Part model, mm, in its own coordinate system. A direction names the side the tool comes from. Coordinates: 2 decimals unless noted, no trailing zeros. Write each loop counter-clockwise with the first axis right and the second up, starting at its lowest first coordinate (ties: lowest second). Pieces come first, ordered by that corner, then holes. Notation, with made-up numbers: (57.5, -29) - (61.5, -29) arc R25 cw to (61.5, -13) - close; hole circle Ø8 at (61, 24.5). An arc over 180 degrees is marked (long way). Write each question's results on one line, items separated by ' | '.
from build123d import *

# Parameters (mm, degrees)
SKETCH1_R           = 3.7084
SKETCH1_W           = 1.778
SKETCH1_H           = 1.5875
SKETCH1_W_2         = 1.5875
SKETCH1_H_2         = 1.3208
BOSS_EXTRUDE1_DEPTH = 1.5875
SKETCH3_W           = 3.683
SKETCH3_H           = 3.302
CUT_EXTRUDE1_DEPTH  = 23.34938408
FILLET1_R           = 1.27


with BuildPart() as part:
    # Sketch1 → Boss-Extrude1 (new body)
    # profile 1 of 4: a face of its own
    with BuildSketch(Plane.XY):
        with BuildLine():
            Line((-10.431265191, -4.028360607), (-2.823309713, -4.028360607))
            Line((-2.823309713, -4.028360607), (12.7, -2.670246987))
            Line((12.7, -2.670246987), (12.7, 16.51))
            Line((12.7, 16.51), (10.10362126, 16.51))
            Line((10.10362126, 16.51), (8.32562126, 16.51))
            Line((8.32562126, 16.51), (-4.89637874, 16.51))
            Line((-4.89637874, 16.51), (-6.67437874, 16.51))
            Line((-6.67437874, 16.51), (-7.62, 16.51))
            ThreePointArc((-7.62, 16.51), (-10.314076836, 15.394076836), (-11.43, 12.7))
            Line((-11.43, 12.7), (-11.43, 1.3208))
            Line((-11.43, 1.3208), (-11.43, 0))
            Line((-11.43, 0), (-11.43, -2.009424845))
            ThreePointArc((-11.43, -2.009424845), (-11.166665718, -3.135654487), (-10.431265191, -4.028360607))
        make_face()
        Circle(SKETCH1_R, mode=Mode.SUBTRACT)
        with BuildLine():
            ThreePointArc((-3.82905, 11.642311449), (4.572, 9.144), (-3.82905, 6.645688551))
            ThreePointArc((-3.82905, 6.645688551), (-7.874, 9.144), (-3.82905, 11.642311449))
        make_face(mode=Mode.SUBTRACT)
    # profile 2 of 4: a face of its own
    with BuildSketch(Plane.XY):
        with Locations((-5.78537874, 17.30375)):
            Rectangle(SKETCH1_W, SKETCH1_H)
    # profile 3 of 4: a face of its own
    with BuildSketch(Plane.XY):
        with Locations((9.21462126, 17.30375)):
            Rectangle(SKETCH1_W, SKETCH1_H)
    # profile 4 of 4: a face of its own
    with BuildSketch(Plane.XY):
        with Locations((-12.22375, 0.6604)):
            Rectangle(SKETCH1_W_2, SKETCH1_H_2)
    extrude(amount=BOSS_EXTRUDE1_DEPTH)

    # Sketch3 → Cut-Extrude1 (cut, through all)
    with BuildSketch(Plane.XY.offset(1.5875)):
        with Locations((5.753177383, 14.859)):
            Rectangle(SKETCH3_W, SKETCH3_H)
    extrude(amount=-CUT_EXTRUDE1_DEPTH, mode=Mode.SUBTRACT)

    # Fillet1
    fillet1_edges = [part.edges().sort_by_distance(p)[0] for p in [
        (7.594677383, 13.208, 0.79375),
        (3.911677383, 13.208, 0.79375),
    ]]
    fillet(fillet1_edges, radius=FILLET1_R)


solid = part.part
(1) 3-axis set-ups, long thin cutter, end or side, ignore diameter. For faces 4 (the flat face through (11, 16.51, 1)), 5 (the flat face through (3.912, 15, 1)), 6 (the flat face through (-12, 1.321, 1)): which of +Z, -Z, +X, -X, +Y, -Y reach the whole face in a straight line?
Return value:
face 4: +Z, -Z, +X, +Y | face 5: +Z, -Z, +Y | face 6: +Z, -Z, -X, +Y
(2) Flat gauge pins, fed straight in: P1, Ø0.9, axis at x = 5.5, z = 0.5, coming from the +Y side; P2, Ø0.5, axis at y = 16, z = 0.5, coming from the -X side; P3, Ø6.5, axis at x = 0, y = 0, coming from the -Z side. Where does each tip first touch, or does it go through?
Return value:
P1: stops at y = 13.21 | P2: stops at x = -9.9 | P3: passes through
(3) Saw through at D-D on x = 2.25. Write the cut outline in (y, z), then the cut area to 3 significant figures.
Return value:
outline: (-3.58, 0) - (-2.95, 0) - (-2.95, 1.59) - (-3.58, 1.59) - close; (2.95, 0) - (5.16, 0) - (5.16, 1.59) - (2.95, 1.59) - close; (13.12, 0) - (16.51, 0) - (16.51, 1.59) - (13.12, 1.59) - close | area: 9.90 mm^2
(4) Wall check: line 1 (X direction, y = 17, z = 0.65); line 2 (Y direction, x = 1.5, z = 0.7); line 3 (Y direction, x = -5.08, z = 0.7). Give the ranges that are in metal, low to high. Write a range as from..to.
Return value:
line 1: x = -6.67..-4.9, 8.33..10.1 | line 2: y = -3.65..-3.39, 3.39..4.83, 13.46..16.51 | line 3: y = -4.03..6.35, 11.94..18.1
(5) Saw through at A-A on y = 2.25. Write the cut outline in (x, z).
Return value:
outline: (-11.43, 0) - (-2.95, 0) - (-2.95, 1.59) - (-11.43, 1.59) - close; (2.95, 0) - (12.7, 0) - (12.7, 1.59) - (2.95, 1.59) - close
(6) Saw through at B-B on x = -6. Write the cut outline in (y, z), then the cut area to 3 significant figures.
Return value:
outline: (-4.03, 0) - (6.51, 0) - (6.51, 1.59) - (-4.03, 1.59) - close; (11.78, 0) - (18.1, 0) - (18.1, 1.59) - (11.78, 1.59) - close | area: 26.7 mm^2
(7) Saw through at C-C on z = 1.15. Write the cut outline in (x, y).
Return value:
outline: (-13.02, 0) - (-11.43, 0) - (-11.43, -2.01) arc R2.54 ccw to (-10.43, -4.03) - (-2.82, -4.03) - (12.7, -2.67) - (12.7, 16.51) - (10.1, 16.51) - (10.1, 18.1) - (8.33, 18.1) - (8.33, 16.51) - (7.59, 16.51) - (7.59, 14.48) arc R1.27 cw to (6.32, 13.21) - (5.18, 13.21) arc R1.27 cw to (3.91, 14.48) - (3.91, 16.51) - (-4.9, 16.51) - (-4.9, 18.1) - (-6.67, 18.1) - (-6.67, 16.51) - (-7.62, 16.51) arc R3.81 ccw to (-11.43, 12.7) - (-11.43, 1.32) - (-13.02, 1.32) - close; hole (-3.83, 6.65) arc R4.57 ccw (long way) to (-3.83, 11.64) arc R2.79 ccw (long way) to start; hole circle Ø7.42 at (0, 0)
(8) Two-plate mould, pull along Y, no slides. Class faces 1 (the flat face through (6, 13.208, 1)), 2 (the cylindrical face through (1.71, -3.29, 0.78)), 3 (the flat face through (10.104, 17, 1)): released by +Y, released by -Y, zero draft, split by the parting line, or undercut.
Return value:
face 1: released by +Y | face 2: undercut | face 3: zero draft
